```python
from build123d import *

# Parameters (mm, degrees)
SKETCH2_R           = 2
BOSS_EXTRUDE1_DEPTH = 60
BOSS_EXTRUDE2_DEPTH = 2.8
SKETCH5_OUTSIDE_W   = 33.75
SKETCH5_OUTSIDE_H   = 34.832
SKETCH5_OUTSIDE_R   = 3.325
CUT_EXTRUDE1_DEPTH  = 2.8
CUT_EXTRUDE1_DRAFT  = -65
FILLET7_R           = 0.14
CHAMFER1_SIZE       = 0.525
FILLET4_R           = 0.1
CUT_EXTRUDE2_START  = -42.5
SKETCH6_R           = 2
CUT_EXTRUDE2_DEPTH  = 42.5


with BuildPart() as part:
    # Sketch2 → Boss-Extrude1 (new body)
    with BuildSketch(Plane(origin=(0, 0, 0), x_dir=(0, 0, -1), z_dir=(1, 0, 0))):
        Circle(SKETCH2_R)
    extrude(amount=BOSS_EXTRUDE1_DEPTH)

    # Sketch3 → Boss-Extrude2 (add)
    with BuildSketch(Plane.ZY):
        Polygon((0, 4.041451884), (-3.5, 2.020725942), (-3.5, -2.020725942), (0, -4.041451884), (3.5, -2.020725942), (3.5, 2.020725942), align=None)
    extrude(amount=BOSS_EXTRUDE2_DEPTH)


with BuildPart() as cut_extrude1_tool:
    # Sketch5 outside → Cut-Extrude1 (with draft: the straight prism first)
    with BuildSketch(Plane.ZY.offset(2.8)):
        Rectangle(SKETCH5_OUTSIDE_W, SKETCH5_OUTSIDE_H)
        Circle(SKETCH5_OUTSIDE_R, mode=Mode.SUBTRACT)
    extrude(amount=-CUT_EXTRUDE1_DEPTH)
    # Cut-Extrude1: the draft: its side faces are tilted about the plane it starts from
    cut_extrude1_sides = [cut_extrude1_tool.faces().sort_by_distance(p)[0] for p in [
        (-1.4, -17.416, 0),
        (-1.4, 0, 16.875),
        (-1.4, 17.416, 0),
        (-1.4, 0, -16.875),
        (-1.4, 0, -3.325),
    ]]
    draft(cut_extrude1_sides, Plane.ZY.offset(2.8), CUT_EXTRUDE1_DRAFT)


with BuildPart() as part_1:
    add(part.part)

    # Cut-Extrude1: cut by cut_extrude1_tool
    add(cut_extrude1_tool.part, mode=Mode.SUBTRACT)

    # Fillet7
    fillet7_edges = [part_1.edges().sort_by_distance(p)[0] for p in [
        (-1.2329565, -4.041451884, 0),
        (-1.2329565, -2.020725942, -3.5),
        (-1.2329565, 2.020725942, -3.5),
        (-1.2329565, 4.041451884, 0),
        (-1.2329565, -2.020725942, 3.5),
        (-1.2329565, 2.020725942, 3.5),
    ]]
    fillet(fillet7_edges, radius=FILLET7_R)

    # Chamfer1
    chamfer1_edges = [part_1.edges().sort_by_distance(p)[0] for p in [
        (60, 0, 2),
    ]]
    chamfer(chamfer1_edges, length=CHAMFER1_SIZE)

    # Fillet4
    fillet4_edges = [part_1.edges().sort_by_distance(p)[0] for p in [
        (0, 0, 2),
    ]]
    fillet(fillet4_edges, radius=FILLET4_R)

    # Sketch6 → Cut-Extrude2 (cut)
    with BuildSketch(Plane(origin=(60, 0, 0), x_dir=(0, 0, -1), z_dir=(1, 0, 0)).offset(CUT_EXTRUDE2_START)):
        with Locations(Location((0, 0, 0), (0, 0, 180))):
            Circle(SKETCH6_R)
    extrude(amount=CUT_EXTRUDE2_DEPTH, mode=Mode.SUBTRACT)


solid = part_1.part
```
The model under review builds one solid part; all positions refer to its coordinate system, in mm. A direction names the side the tool comes from. Give positions to 0.01 mm unless a question says otherwise; leave off trailing zeros. Write each loop counter-clockwise with the first axis right and the second up, starting at its lowest first coordinate (ties: lowest second). Pieces come first, ordered by that corner, then holes. Notation, with made-up numbers: M -25,-17 L 8,-17 A12 ccw 8,-3 Z; hole C 24,18.25 d5. An arc over 180 degrees is marked long. Write item = value, one per line. Start each with the question number.
Q1. For line 1 (X direction, y = 0, z = -3); line 2 (Y direction, x = 11, z = -0.5); line 3 (Y direction, x = 6.25, z = 0), list the stretches that pass through material, from the lowest coordinate up.
Q2. We need section A-A (y = 0). State the section outline as (x, z) points (3 decimals), plus the area to 3 significant figures.
Q3. Machinability: for faces 1 (the face through (-1, 0, 3.5)), 2 (the face through (0, -2, -2)), which of the approach directions +Z, -Z, +X, -X, +Y, -Y give a long, thin tool a straight path to every point of the face, cutting with its end or side? Answer none if there is none.
Q4. Clearance check with flat-ended pins moving along their axes: pin 1 (3 mm diameter, centred on x = 10.5, z = 1, fed in from +Y); pin 2 (1 mm diameter, centred on x = 11.5, z = -1, fed in from -Y); pin 3 (1.5 mm diameter, centred on x = 1.5, y = -2.5, fed in from +Z). State where each tip first meets the part, or that it passes through.
Q5. We need section B-B (x = 0.5). State the section outline as (y, z) points, plus the area to 3 significant figures.
Result set:
q1.line_1 = -2.8 to 0
q1.line_2 = -1.94 to 1.94
q1.line_3 = -2 to 2
q2.outline = M -2.8,-3.325 L -2.718,-3.5 L 0,-3.5 L 0,-2.1 A0.1 cw 0.1,-2 L 17.5,-2 L 17.5,2 L 0.1,2 A0.1 cw 0,2.1 L 0,3.5 L -2.718,3.5 L -2.8,3.325 Z
q2.area = 89.6 mm2
q3.face_1 = +Z, +X, -X, +Y, -Y
q3.face_2 = +X
q4.pin_1 = 2
q4.pin_2 = -1.94
q4.pin_3 = 0.97
q5.outline = C 0,0 d4
q5.area = 12.6 mm2
